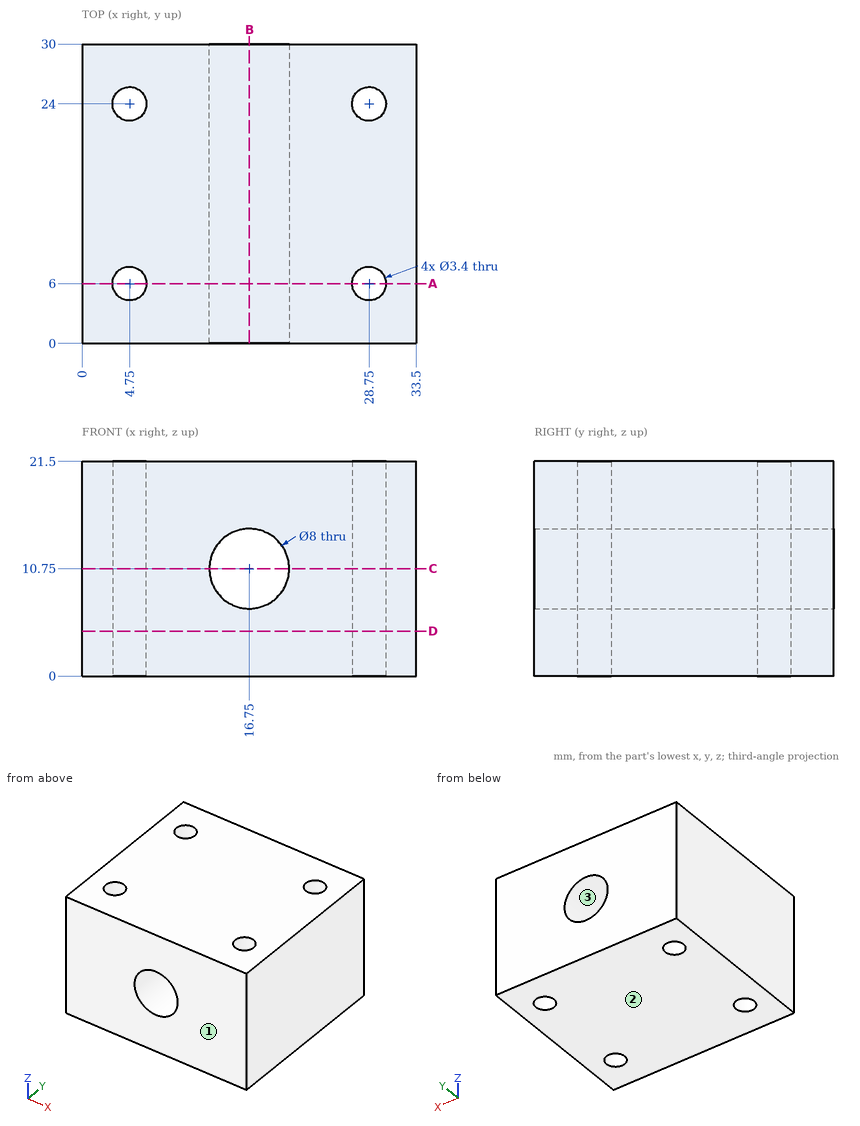
Input: dimensioned drawing with shaded views. Units: mm. Origin: part minimum x, y, z. Give positions to 0.01 mm unless a question says otherwise; leave off trailing zeros. Write each loop counter-clockwise with the first axis right and the second up, starting at its lowest first coordinate (ties: lowest second). Pieces come first, ordered by that corner, then holes.
1. Section query A-A, the plane y = 6. Return loops of the section in (x, z), then the cut area to 3 significant figures.
2. Pin query (flat end, axial travel): P1, Ø2, axis at x = 4.75, y = 24, coming from the +Z side; P2, Ø4, axis at x = 28.75, y = 24, coming from the -Z side. Return the tip coordinate at first contact, or that it passes through.
3. Section query C-C, the plane z = 10.75. Return loops of the section in (x, y).
4. Section query D-D, the plane z = 4.5. Return loops of the section in (x, y).
5. Draft query along Z for the marked faces 1, 2 and 3. Return one class per face: released by +Z, released by -Z, zero draft, split by the parting line, or undercut.
6. Section query B-B, the plane x = 16.75. Return loops of the section in (y, z), then the cut area to 3 significant figures.
7. Line query: probe 1 along Y at (x, z) = (28.75, 14); probe 2 along X at (y, z) = (24, 15.75); probe 3 along X at (y, z) = (11.75, 11). Output: solid intervals per line, ascending.
Computed:
1. outline: (0, 0) - (3.05, 0) - (3.05, 21.5) - (0, 21.5) - close; (6.45, 0) - (27.05, 0) - (27.05, 21.5) - (6.45, 21.5) - close; (30.45, 0) - (33.5, 0) - (33.5, 21.5) - (30.45, 21.5) - close; hole circle Ø8 at (16.75, 10.75)
1. area: 524 mm2
2. P1: passes through
2. P2: stops at z = 0
3. outline: (0, 0) - (12.75, 0) - (12.75, 30) - (0, 30) - close; (20.75, 0) - (33.5, 0) - (33.5, 30) - (20.75, 30) - close; hole circle Ø3.4 at (4.75, 6); hole circle Ø3.4 at (4.75, 24); hole circle Ø3.4 at (28.75, 6); hole circle Ø3.4 at (28.75, 24)
4. outline: (0, 0) - (33.5, 0) - (33.5, 30) - (0, 30) - close; hole circle Ø3.4 at (4.75, 6); hole circle Ø3.4 at (4.75, 24); hole circle Ø3.4 at (28.75, 6); hole circle Ø3.4 at (28.75, 24)
5. face 1: zero draft
5. face 2: released by -Z
5. face 3: undercut
6. outline: (0, 0) - (30, 0) - (30, 6.75) - (0, 6.75) - close; (0, 14.75) - (30, 14.75) - (30, 21.5) - (0, 21.5) - close
6. area: 405 mm2
7. probe 1: y = 0 to 4.3, 7.7 to 22.3, 25.7 to 30
7. probe 2: x = 0 to 3.05, 6.45 to 27.05, 30.45 to 33.5
7. probe 3: x = 0 to 12.76, 20.74 to 33.5
